The listing builds one solid part. Answer for the finished solid, in the listing's coordinates (mm). A direction names the side the tool comes from. Round coordinates to 2 decimals unless told otherwise and drop trailing zeros. Loops run counter-clockwise (first coordinate to the right, second up) from the corner with the lowest first, then second, coordinate; pieces in that order, holes last. Notation, with made-up numbers: (24, 67) -> (29, 67) arc R29 ccw to (29, 105) -> close; hole circle Ø11 at (81.25, -3.75). An arc over 180 degrees is marked (long way). Answer in a Markdown table with one row per item. Add a question column.
Autodesk Inventor part; units mm, degrees
ref_plane "YZ Plane" through (0, 0, 0) normal (1, 0, 0) x (0, 1, 0)
ref_plane "XZ Plane" through (0, 0, 0) normal (0, 1, 0) x (-1, 0, 0)
ref_plane "XY Plane" through (0, 0, 0) normal (0, 0, 1) x (1, 0, 0)
sketch "Sketch1" plane through (0, 0, 0) normal (0, 1, 0) x (-1, 0, 0)
  circle A0 centre (0.4121, -148.477) radius 4
  arc A1 (9.1115, -162.2046) -> (9.3712, -161.5303) centre (7.8828, -161.3443) ccw
  line L0 (9.1115, -162.2046) -> (4.9561, -168.1392)
  arc A2 (2.867, -168.5075) -> (4.9561, -168.1392) centre (3.7274, -167.2788) ccw
  line L1 (2.867, -168.5075) -> (-9.0439, -160.1674)
  arc A3 (-9.6719, -159.1247) -> (-9.0439, -160.1674) centre (-8.1835, -158.9387) ccw
  line L2 (-9.6719, -159.1247) -> (-12.2297, -138.6622)
  arc A4 (-12.5, -134.321) -> (-12.2297, -138.6622) centre (22.5, -134.321) ccw
  line L3 (-12.5, -134.321) -> (-12.5, -23.3333)
  arc A5 (-12.5, -23.3333) -> (-14.5, -17.3333) centre (-22.5, -23.3333) ccw
  line L4 (-14.5, -17.3333) -> (-18, -12.6667)
  arc A6 (-20, -6.6667) -> (-18, -12.6667) centre (-10, -6.6667) ccw
  line L5 (-20, -6.6667) -> (-20, 5.4953)
  arc A7 (-16.6262, 12.9849) -> (-20, 5.4953) centre (-10, 5.4953) ccw
  line L6 (-16.6262, 12.9849) -> (-6.6262, 21.8321)
  arc A8 (6.6262, 21.8321) -> (-6.6262, 21.8321) centre (0, 14.3426) ccw
  line L7 (6.6262, 21.8321) -> (16.6262, 12.9849)
  arc A9 (20, 5.4953) -> (16.6262, 12.9849) centre (10, 5.4953) ccw
  line L8 (20, 5.4953) -> (20, -6.6667)
  arc A10 (18, -12.6667) -> (20, -6.6667) centre (10, -6.6667) ccw
  line L9 (18, -12.6667) -> (14.5, -17.3333)
  arc A11 (14.5, -17.3333) -> (12.5, -23.3333) centre (22.5, -23.3333) ccw
  line L10 (12.5, -23.3333) -> (12.5, -134.321)
  arc A12 (12.2297, -138.6622) -> (12.5, -134.321) centre (-22.5, -134.321) ccw
  line L11 (12.2297, -138.6622) -> (9.3712, -161.5303)
  arc A13 (-7.7782, -5.6569) -> (-5.6569, -7.7782) centre (-6.7175, -6.7175) ccw
  line L12 (-7.7782, -5.6569) -> (-6.7175, -4.5962)
  arc A14 (-4.5962, -6.7175) -> (-6.7175, -4.5962) centre (-5.6569, -5.6569) ccw
  line L13 (-4.5962, -6.7175) -> (-5.6569, -7.7782)
  circle A15 centre (-6, -136.5) radius 1.5
  circle A16 centre (6, -136.5) radius 1.5
  arc A17 (5.6569, -7.7782) -> (7.7782, -5.6569) centre (6.7175, -6.7175) ccw
  line L14 (5.6569, -7.7782) -> (4.5962, -6.7175)
  arc A18 (6.7175, -4.5962) -> (4.5962, -6.7175) centre (5.6569, -5.6569) ccw
  line L15 (6.7175, -4.5962) -> (7.7782, -5.6569)
  circle A19 centre (0, -124.0736) radius 1.5
  line L16 (6.7175, 4.5962) -> (7.7782, 5.6569)
  arc A20 (7.7782, 5.6569) -> (5.6569, 7.7782) centre (6.7175, 6.7175) ccw
  line L17 (5.6569, 7.7782) -> (4.5962, 6.7175)
  arc A21 (4.5962, 6.7175) -> (6.7175, 4.5962) centre (5.6569, 5.6569) ccw
  circle A22 centre (0, 0) radius 3
  arc A23 (-6.7175, 4.5962) -> (-4.5962, 6.7175) centre (-5.6569, 5.6569) ccw
  line L18 (-6.7175, 4.5962) -> (-7.7782, 5.6569)
  arc A24 (-5.6569, 7.7782) -> (-7.7782, 5.6569) centre (-6.7175, 6.7175) ccw
  line L19 (-5.6569, 7.7782) -> (-4.5962, 6.7175)
  point P0 (12.5, -23.3333)
  point P1 (14.5, -17.3333)
  point P2 (16.6262, 12.9849)
  point P3 (6.6262, 21.8321)
  point P4 (-6.6262, 21.8321)
  point P5 (-18, -12.6667)
  point P6 (-12.5, -23.3333)
  point P7 (4.9561, -168.1392)
  point P8 (7.7782, -5.6569)
  point P9 (5.6569, -7.7782)
  point P10 (4.5962, -6.7175)
  point P11 (6.7175, 4.5962)
  point P12 (-7.7782, 5.6569)
  point P13 (-5.6569, 7.7782)
  point P14 (-4.5962, -6.7175)
  point P15 (-5.6569, -7.7782)
extrude "Extrusion1" add sketch "Sketch1" along normal blind 6
sketch "Sketch2" plane through (0, 6, 0) normal (0, 1, 0) x (1, 0, 0)
  circle A0 centre (0, 124.0736) radius 1.5 construction
  circle A1 centre (-0.4121, 148.477) radius 4 construction
  point P0 (0, 0)
properties part number "og kauri arm"
Item 1: Section A-A, the plane z = 0 is taken. Write down the section's boundary in (x, y).
Item 2: For faces 5 (the flat face through (12.5, 3, -80)), 6 (the cylindrical face through (19.14, 2.96, 9.55)), determine the directions among +Z, -Z, +X, -X, +Y, -Y from which every point of the face is accessible in a straight line to the end or side of a thin tool.
Item 3: Consider L1, parallel to Z at x = 0, y = 2.8; L2, parallel to Z at x = -6, y = 1.9; L3, parallel to X at y = 0.75, z = -75.5. Determine where each line is inside the solid, lowest interval first. Write a range as from..to.
Item 4: Section B-B, the plane y = 4.4 is taken. Give the number of separate pieces and of enclosed holes in the cut face, and give its area (3 significant figures).
Item 5: Flat-ended cylindrical pins translate along their axes: P1, Ø3, axis at y = 4, z = -85, coming from the +X side; P2, Ø1, axis at x = -15.5, y = 5, coming from the -Z side; P3, Ø3, axis at y = 4.5, z = -24.5, coming from the -X side. Find the tip coordinate at first contact, or state that the pin passes through.
Item 6: Section C-C, the plane z = -82.5 is taken. Write down the section's boundary in (x, y), and give its area (3 significant figures).
Item 7: The mould has two halves that part along Z. Classify faces 1 (the cylindrical face through (13.028, 2.958, -20.128)), 2 (the cylindrical face through (0.455, 2.958, -144.572)), 3 (the cylindrical face through (0.101, 2.958, 24.342)), 4 (the cylindrical face through (0.33, 2.96, -122.61)): +Z half, -Z half, draft (parallel to the pull), parting line (faces both ways), or undercut.
Here are the results:
| question | item | result |
|---|---|---|
| 1 | outline | (-20, 0) -> (-3, 0) -> (-3, 6) -> (-20, 6) -> close; (3, 0) -> (20, 0) -> (20, 6) -> (3, 6) -> close |
| 2 | face 5 | -Z, +X, +Y, -Y |
| 2 | face 6 | +Z, +X, +Y, -Y |
| 3 | L1 | z = -166.5..-152.46, -144.5..-125.57, -122.57..-3, 3..24.34 |
| 3 | L2 | z = -166.65..-138, -135..-8.03, -4.2..4.2, 8.03..22.34 |
| 3 | L3 | x = -12.5..12.5 |
| 4 | separate pieces | 1 |
| 4 | enclosed holes | 9 |
| 4 | area | 4,830 mm² |
| 5 | P1 | stops at x = 12.5 |
| 5 | P2 | stops at z = -16.67 |
| 5 | P3 | stops at x = -12.51 |
| 6 | outline | (-12.5, 0) -> (12.5, 0) -> (12.5, 6) -> (-12.5, 6) -> close |
| 6 | area | 150 mm² |
| 7 | face 1 | -Z half |
| 7 | face 2 | undercut |
| 7 | face 3 | +Z half |
| 7 | face 4 | undercut |
